from build123d import *

# Parameters (mm, degrees)
F0_R          = 18
F0_R_2        = 15
F1_DEPTH      = 28
F3_DEPTH      = 20
F4_DEPTH      = 20
F5_R          = 9
F6_DEPTH      = 25
F7_R          = 17
F7_R_2        = 6.5
F8_DEPTH      = 20
F9_SIZE2      = 2
F9_SIZE       = 0.5
F10_DEPTH     = 20
F11_W         = 10
F11_H         = 20
F12_DEPTH     = 17
F13_R         = 15
F14_DEPTH     = 30
F15_R         = 7
F16_DEPTH     = 200
F17_T4_ANGLE  = 187.4641783336
F17_S5_R      = 17
F17_T6_DEPTH  = 27
F17_T11_ANGLE = 187.4641783336
F17_S12_R     = 17
F17_T13_DEPTH = 27
F18_R         = 10.25
F18_R_2       = 7
F19_DEPTH     = 25
F20_R         = 6
F21_DEPTH     = 45


# Not quite as in the source:
# - a fillet or chamfer that OpenCascade refuses, or shapes differently, is made with other operations: its cross-section is extruded or revolved along the edge and cut away or added


with BuildPart() as f1:
    # F0 (on Front) → F1 (new body)
    with BuildSketch(Plane.XZ):
        Circle(F0_R)
        Circle(F0_R_2, mode=Mode.SUBTRACT)
    extrude(amount=F1_DEPTH)

    # F2 (on Right) → F3 (join)
    with BuildSketch(Plane.YZ):
        Polygon((0, -8), (0, 0), (0, 8), (-28, 8), (-28, -8), align=None)
    extrude(amount=-F3_DEPTH)

    # F4 (add): a face of the model
    f4_faces = [f1.faces().sort_by_distance(p)[0] for p in [
        (0, -14, 0),
    ]]
    extrude(f4_faces, amount=F4_DEPTH)

    # F5 (on face) → F6 (cut)
    with BuildSketch(Plane.XZ.offset(28)):
        Circle(F5_R)
    extrude(amount=-F6_DEPTH, mode=Mode.SUBTRACT)

    # F7 (on face) → F8 (join)
    with BuildSketch(Plane(origin=(0, 0, 0), x_dir=(-1, 0, 0), z_dir=(0, 1, 0))):
        Circle(F7_R)
        Circle(F7_R_2, mode=Mode.SUBTRACT)
    extrude(amount=F8_DEPTH)

    # F9
    f9_edges = [f1.edges().sort_by_distance(p)[0] for p in [
        (17, 20, 0),
    ]]
    f9_side = f1.faces().sort_by_distance((16.519167, 20, 0))[0]
    chamfer(f9_edges, length=F9_SIZE, length2=F9_SIZE2, reference=f9_side)

    # F10 (add): a face of the model
    f10_faces = [f1.faces().sort_by_distance(p)[0] for p in [
        (16.0333095244, 20, 0),
    ]]
    extrude(f10_faces, amount=F10_DEPTH)

    # F11 (on Top) → F12 (join)
    with BuildSketch(Plane.XY):
        with Locations((-5, 30)):
            Rectangle(F11_W, F11_H)
        with Locations((5, 30)):
            Rectangle(F11_W, F11_H)
    extrude(amount=F12_DEPTH)

    # F13 (on face) → F14 (cut)
    with BuildSketch(Plane.XZ.offset(28)):
        Circle(F13_R)
    extrude(amount=-F14_DEPTH, mode=Mode.SUBTRACT)

    # F15 (on face) → F16 (cut)
    with BuildSketch(Plane(origin=(0, 40, 0), x_dir=(-1, 0, 0), z_dir=(0, 1, 0))):
        Circle(F15_R)
        with BuildLine():
            Line((-6.5, 0), (6.5, 0))
            ThreePointArc((6.5, 0), (0, -6.5), (-6.5, 0))
        make_face(mode=Mode.SUBTRACT)
    extrude(amount=-F16_DEPTH, mode=Mode.SUBTRACT)

    # F17: chamfer of 3 x 2 on 2 edges, made by hand


with BuildPart() as f17_tool2:
    # F17_s3 → F17_t4 (revolve)
    with BuildSketch(Plane(origin=(0, 0, 0), x_dir=(0, 1, 0), z_dir=(0.0650911923, 0, 0.9978793197))):
        with BuildLine():
            Line((0.7488452649, 15.5007698234), (-3.7488452649, 18.4992301766))
            Line((-3.7488452649, 18.4992301766), (-3.7488452649, 18.9492301766))
            ThreePointArc((-3.7488452649, 18.9492301766), (-1.8744226325, 18.45), (0, 18.45))
            Line((0, 18.45), (0.45, 18))
            ThreePointArc((0.45, 18), (0.45, 16.7503849117), (1.1988452649, 15.5007698234))
            Line((1.1988452649, 15.5007698234), (0.7488452649, 15.5007698234))
        make_face()
    revolve(axis=Axis((0, 0, 0), (0, -1, 0)), revolution_arc=F17_T4_ANGLE)

    # F17_s5 → F17_t6 (cut, symmetric)
    with BuildSketch(Plane.XZ.offset(0.9)):
        Circle(F17_S5_R)
    extrude(amount=F17_T6_DEPTH, both=True, mode=Mode.SUBTRACT)

    split(bisect_by=Plane.XY.offset(-8), keep=Keep.BOTTOM)


with BuildPart() as f1_1:
    add(f1.part)

    # F17_t1: cut F17_tool2
    add(f17_tool2.part, mode=Mode.SUBTRACT)


with BuildPart() as f17_tool9:
    # F17_s10 → F17_t11 (revolve)
    with BuildSketch(Plane(origin=(0, 0, 0), x_dir=(0, 1, 0), z_dir=(-0.0650911923, 0, -0.9978793197))):
        with BuildLine():
            Line((0.7488452649, 15.5007698234), (-3.7488452649, 18.4992301766))
            Line((-3.7488452649, 18.4992301766), (-3.7488452649, 18.9492301766))
            ThreePointArc((-3.7488452649, 18.9492301766), (-1.8744226325, 18.45), (0, 18.45))
            Line((0, 18.45), (0.45, 18))
            ThreePointArc((0.45, 18), (0.45, 16.7503849117), (1.1988452649, 15.5007698234))
            Line((1.1988452649, 15.5007698234), (0.7488452649, 15.5007698234))
        make_face()
    revolve(axis=Axis((0, 0, 0), (0, -1, 0)), revolution_arc=F17_T11_ANGLE)

    # F17_s12 → F17_t13 (cut, symmetric)
    with BuildSketch(Plane.XZ.offset(0.9)):
        Circle(F17_S12_R)
    extrude(amount=F17_T13_DEPTH, both=True, mode=Mode.SUBTRACT)

    split(bisect_by=Plane.XY.offset(8), keep=Keep.TOP)


with BuildPart() as f1_2:
    add(f1_1.part)

    # F17_t8: cut F17_tool9
    add(f17_tool9.part, mode=Mode.SUBTRACT)

    # F18 (on face) → F19 (join)
    with BuildSketch(Plane(origin=(0, 40, 0), x_dir=(-1, 0, 0), z_dir=(0, 1, 0))):
        Circle(F18_R)
        Circle(F18_R_2, mode=Mode.SUBTRACT)
    extrude(amount=F19_DEPTH)

    # F20 (on face) → F21 (cut)
    with BuildSketch(Plane(origin=(-20, 0, 0), x_dir=(0, -1, 0), z_dir=(-1, 0, 0))):
        with Locations((14, 0)):
            Circle(F20_R)
    extrude(amount=-F21_DEPTH, mode=Mode.SUBTRACT)


solid = f1_2.part
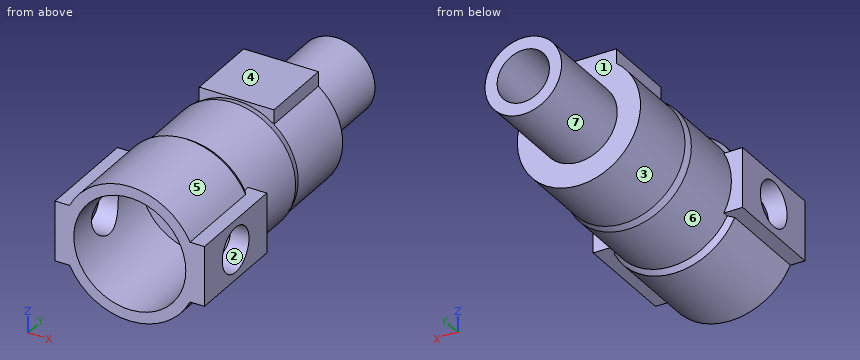
Work out the finished part from the listing and answer in its coordinate system (mm). Face numbers are marked on the shaded views. A direction names the side the tool comes from. Give positions to 0.01 mm unless a question says otherwise; leave off trailing zeros. Loops run counter-clockwise (first coordinate to the right, second up) from the corner with the lowest first, then second, coordinate; pieces in that order, holes last. Notation, with made-up numbers: (23, 20) -> (82, 20) arc R19 ccw to (82, 32) -> close; hole circle Ø8 at (-15.75, 73). An arc over 180 degrees is marked (long way). Use a Markdown table: item, result. Add a question column.
1. Flat-ended cylindrical pins translate along their axes: pin 1 Ø16 at (x, y) = (-1.5, 30.5) entering from +Z; pin 2 Ø5.5 at (x, y) = (-17.5, -15) entering from +Z; pin 3 Ø9 at (x, z) = (0, -3.5) entering from -Y; pin 4 Ø9.5 at (y, z) = (-14, 0) entering from +X. Find the tip coordinate at first contact, or state that the pin passes through.
2. Section A-A on y = -14 is taken. Determine the outline of the cut face in (x, z).
3. Find the intervals of material crossed by probe 1 along Z at (x, y) = (0, -21); probe 2 along Z at (x, y) = (17, -14); probe 3 along Y at (x, z) = (-16.25, 0), in increasing order.
4. Section B-B on z = 0 is taken. State how many separate pieces and enclosed holes the cut face has, and give its area (3 significant figures).
5. Section D-D on y = 37 is taken. Determine the outline of the cut face in (x, z).
6. Section C-C on x = 0 is taken. Determine the outline of the cut face in (y, z), and give its area (3 significant figures).
7. For the marked faces 4, 5, 6 and 7, determine the directions among +Z, -Z, +X, -X, +Y, -Y from which every point of the face is accessible in a straight line to the end or side of a thin tool.
8. Determine the mould class of the marked faces 1, 2 and 3 for opening direction Z: released by +Z, released by -Z, zero draft, split by the parting line, or undercut.
Results below:
| question | item | result |
|---|---|---|
| 1 | pin 1 | stops at z = 17 |
| 1 | pin 2 | stops at z = 10.32 |
| 1 | pin 3 | stops at y = 2 |
| 1 | pin 4 | passes through |
| 2 | outline | (-20, -8) -> (-16.12, -8) arc R18 ccw to (16.12, -8) -> (20, -8) -> (20, -6) -> (13.75, -6) arc R15 cw to (-13.75, -6) -> (-20, -6) -> close; (-20, 6) -> (-13.75, 6) arc R15 cw to (13.75, 6) -> (20, 6) -> (20, 8) -> (16.12, 8) arc R18 ccw to (-16.12, 8) -> (-20, 8) -> close |
| 3 | probe 1 | z = -18 to -15, 15 to 18 |
| 3 | probe 2 | z = -8 to -6, 6 to 8 |
| 3 | probe 3 | y = -28 to -20, -8 to 40 |
| 4 | separate pieces | 4 |
| 4 | enclosed holes | 0 |
| 4 | area | 1,070 mm^2 |
| 5 | outline | (-10, 13.12) arc R16.5 ccw (long way) to (10, 13.12) -> (10, 17) -> (-10, 17) -> close; hole circle Ø14 at (0, 0) |
| 6 | outline | (-28, -18) -> (-3, -18) -> (-1.5, -17) -> (18, -17) -> (20, -16.5) -> (40, -16.5) -> (40, -10.25) -> (65, -10.25) -> (65, -7) -> (2, -7) -> (2, -15) -> (-28, -15) -> close; (-28, 15) -> (2, 15) -> (2, 7) -> (65, 7) -> (65, 10.25) -> (40, 10.25) -> (40, 17) -> (20, 17) -> (20, 16.5) -> (18, 17) -> (-1.5, 17) -> (-3, 18) -> (-28, 18) -> close |
| 6 | area | 1,080 mm^2 |
| 7 | face 4 | +Z, +X, -X, +Y |
| 7 | face 5 | +Z, -Y |
| 7 | face 6 | none |
| 7 | face 7 | +Y |
| 8 | face 1 | zero draft |
| 8 | face 2 | undercut |
| 8 | face 3 | split by the parting line |
